Design review of the part built by this model. Coordinates are the model's own, in mm. A direction names the side the tool comes from. Round coordinates to 2 decimals unless told otherwise and drop trailing zeros. Loops run counter-clockwise (first coordinate to the right, second up) from the corner with the lowest first, then second, coordinate; pieces in that order, holes last. Notation, with made-up numbers: (-38.5, -11) -> (15.5, -11) arc R20 ccw to (15.5, 7) -> close; hole circle Ø11 at (56.25, 14.5). An arc over 180 degrees is marked (long way). Answer as CSV lines item,"result". Start each with the question number.
(1) Take a section at D-D, the plane z = 0. Write out the cut boundary in (x, y), and give its area (3 significant figures).
(2) Take a section at C-C, the plane y = 9. Write out the cut boundary in (x, z).
(3) Machinability: for faces 4 (the face through (0, 60, -30)), 5 (the face through (28.5, -30, -13)), 6 (the face through (0, 60, 30)), 7 (the face through (0, 62, 25.4)), 8 (the face through (-29.26, 9.76, -31)), which of the approach directions +Z, -Z, +X, -X, +Y, -Y give a long, thin tool a straight path to every point of the face, cutting with its end or side? Answer none if there is none.
(4) Draft analysis for pull direction X (two halves, no side actions). For faces 1 (the face through (29.26, 9.76, -31)), 2 (the face through (-30, 49, 4)), 3 (the face through (25.4, 66, 0)), state which applies: +X half, -X half, draft (parallel to the pull), parting line (faces both ways), or undercut.
(5) To check wall thickness, follow line 1 (Y direction, x = -29.1, z = 0); line 2 (X direction, y = 57, z = 17). State the ranges of each line that lie inside material, in increasing order. Write a range as from..to.
(6) Take a section at B-B, the plane z = 40. Write out the cut boundary in (x, y).
(7) Take a section at A-A, the plane x = 16. Write out the cut boundary in (y, z), and give its area (3 significant figures).
(8) For P1, Ø10, axis at x = -8, z = 1, coming from the -Y side; P2, Ø18.5, axis at x = -10, y = 56, coming from the +Z side; P3, Ø8, axis at x = 4, z = 2.5, coming from the +Y side; P4, Ø12, axis at y = -35, z = -19.5, coming from the -X side, all flat-tipped, find the tip position at first contact; note any pin that passes through.
from build123d import *

# Parameters (mm, degrees)
CROQUIS1_R                   = 50
SALIENTE_EXTRUIR1_DEPTH      = 30
SALIENTE_EXTRUIR2_REACH      = 144.478
SALIENTE_EXTRUIR2_END_RADIUS = 50
CROQUIS3_W                   = 60
CROQUIS3_H                   = 60
CROQUIS3_W_2                 = 50.8
CROQUIS3_H_2                 = 50.8
CROQUIS4_R                   = 45
CROQUIS4_R_2                 = 32.5
CORTAR_EXTRUIR1_DEPTH        = 1.5


with BuildPart() as part:
    # Croquis1 → Saliente-Extruir1 (new, symmetric)
    with BuildSketch(Plane(origin=(0, 0, 0), x_dir=(0, 0, -1), z_dir=(1, 0, 0))):
        Circle(CROQUIS1_R)
    extrude(amount=SALIENTE_EXTRUIR1_DEPTH, both=True)

    # Saliente-Extruir2: up to this cylinder (the profile starts outside it)
    saliente_extruir2_end = Plane(origin=(0, 0, 0), z_dir=(-1, 0, 0)) * Cylinder(SALIENTE_EXTRUIR2_END_RADIUS, 389.956, mode=Mode.PRIVATE)
    # Croquis3 → Saliente-Extruir2 (add, up to the surface)
    with BuildSketch(Plane(origin=(0, 80, 0), x_dir=(1, 0, 0), z_dir=(0, 1, 0)), mode=Mode.PRIVATE) as saliente_extruir2_sk1:
        Rectangle(CROQUIS3_W, CROQUIS3_H)
        Rectangle(CROQUIS3_W_2, CROQUIS3_H_2, mode=Mode.SUBTRACT)
    saliente_extruir2_tool1 = extrude(saliente_extruir2_sk1.sketch, amount=-SALIENTE_EXTRUIR2_REACH, mode=Mode.PRIVATE) - saliente_extruir2_end
    add(saliente_extruir2_tool1.solids().sort_by_distance((0, 80, 29.151472))[0])

    # Croquis4 → Cortar-Extruir1 (cut)
    with BuildSketch(Plane(origin=(30, 0, 0), x_dir=(0, 0, -1), z_dir=(1, 0, 0))):
        Circle(CROQUIS4_R)
        Circle(CROQUIS4_R_2, mode=Mode.SUBTRACT)
    cortar_extruir1 = extrude(amount=-CORTAR_EXTRUIR1_DEPTH, mode=Mode.SUBTRACT)

    # Simetría1: Cortar-Extruir1 across plane
    add(cortar_extruir1.mirror(Plane(origin=(0, 0, 0), x_dir=(0, 0, 1), z_dir=(1, 0, 0))), mode=Mode.SUBTRACT)


solid = part.part
The answers:
1,outline,"(-30, -50) -> (30, -50) -> (30, -45) -> (28.5, -45) -> (28.5, -32.5) -> (30, -32.5) -> (30, 32.5) -> (28.5, 32.5) -> (28.5, 45) -> (30, 45) -> (30, 80) -> (25.4, 80) -> (25.4, 50) -> (-25.4, 50) -> (-25.4, 80) -> (-30, 80) -> (-30, 45) -> (-28.5, 45) -> (-28.5, 32.5) -> (-30, 32.5) -> (-30, -32.5) -> (-28.5, -32.5) -> (-28.5, -45) -> (-30, -45) -> close"
1,area,"6,200 mm²"
2,outline,"(-30, -49.18) -> (30, -49.18) -> (30, -44.09) -> (28.5, -44.09) -> (28.5, -31.23) -> (30, -31.23) -> (30, 31.23) -> (28.5, 31.23) -> (28.5, 44.09) -> (30, 44.09) -> (30, 49.18) -> (-30, 49.18) -> (-30, 44.09) -> (-28.5, 44.09) -> (-28.5, 31.23) -> (-30, 31.23) -> (-30, -31.23) -> (-28.5, -31.23) -> (-28.5, -44.09) -> (-30, -44.09) -> close"
3,face 4,"-Z, +X, -X, +Y"
3,face 5,"+X"
3,face 6,"+Z, +X, -X, +Y"
3,face 7,"+Y"
3,face 8,"-X"
4,face 1,"draft"
4,face 2,"-X half"
4,face 3,"undercut"
5,line 1,"-50..-45, -32.5..32.5, 45..80"
5,line 2,"-30..-25.4, 25.4..30"
6,outline,"(-30, -30) -> (30, -30) -> (30, -20.62) -> (28.5, -20.62) -> (28.5, 20.62) -> (30, 20.62) -> (30, 30) -> (-30, 30) -> (-30, 20.62) -> (-28.5, 20.62) -> (-28.5, -20.62) -> (-30, -20.62) -> close"
7,outline,"(40, -30) -> (80, -30) -> (80, -25.4) -> (43.07, -25.4) arc R50 ccw to (43.07, 25.4) -> (80, 25.4) -> (80, 30) -> (40, 30) arc R50 ccw (long way) to start"
7,area,"8,210 mm²"
8,P1,"y = -50"
8,P2,"z = 30"
8,P3,"y = 50"
8,P4,"x = -30"
